Work out the finished part from the listing and answer in its coordinate system (mm). Face numbers are marked on the shaded views. Coordinates: 2 decimals unless noted, no trailing zeros. Loops run counter-clockwise (first coordinate to the right, second up) from the corner with the lowest first, then second, coordinate; pieces in that order, holes last. Notation, with made-up numbers: (51.25, 9) -> (91.25, 9) arc R12 ccw to (91.25, 31) -> close; hole circle Ø4 at (7, 22). An arc over 180 degrees is marked (long way). Answer as CSV lines item,"result".
Autodesk Inventor part; units mm, degrees
ref_plane "Arbeitsebene1" through (2.5, -44.2, -61.269) normal (-1, 0, 0) x (0, 0, 1)
ref_plane "YZ Plane" through (0, 0, 0) normal (1, 0, 0) x (0, 1, 0)
ref_plane "XZ Plane" through (0, 0, 0) normal (0, 1, 0) x (-1, 0, 0)
sketch "Skizze4" plane through (0, 0, 0) normal (1, 0, 0) x (0, 1, 0)
  line L0 (44.5, 24.853) -> (-44.5, 61.718)
  line L1 (-44.5, 61.718) -> (-44.5, -61.718)
  line L2 (-44.5, -61.718) -> (44.5, -24.853)
  line L3 (44.5, -24.853) -> (44.5, 24.853)
  line L4 (0, -86.4052) -> (0, 86.4052) construction
  line L5 (-62.3, 0) -> (62.3, 0) construction
  dimension "d34" = 89
  dimension "d37" = 112.5
  dimension "d38" = 49.706
extrude "Extrusion2" add sketch "Skizze4" along normal blind 2.5
sketch "Skizze5" plane through (2.5, 0, 0) normal (1, 0, 0) x (0, 0, -1)
  line L0 (-61.718, -44.5) -> (61.718, -44.5) construction
  line L1 (61.718, -44.5) -> (24.853, 44.5) construction
  line L2 (24.853, 44.5) -> (-24.853, 44.5) construction
  line L3 (-24.853, 44.5) -> (-61.718, -44.5) construction
  line L4 (-22.8485, 41.5) -> (22.8485, 41.5)
  line L5 (22.8485, 41.5) -> (57.2282, -41.5)
  line L6 (57.2282, -41.5) -> (-57.2282, -41.5)
  line L7 (-57.2282, -41.5) -> (-22.8485, 41.5)
  line L8 (20.8439, 38.5) -> (-20.8439, 38.5)
  line L9 (-20.8439, 38.5) -> (-52.7384, -38.5)
  line L10 (-52.7384, -38.5) -> (52.7384, -38.5)
  line L11 (52.7384, -38.5) -> (20.8439, 38.5)
  point P0 (0, 0)
  dimension "d8" = 3
  dimension "d9" = 3
extrude "Extrusion3" add sketch "Skizze5" along normal blind 3
sketch "Skizze6" plane through (0, 0, 0) normal (-1, 0, 0) x (0, 0, 1)
  line L0 (24.853, 44.5) -> (-24.853, 44.5) construction
  line L1 (61.718, -44.5) -> (24.853, 44.5) construction
  line L2 (-24.853, 44.5) -> (24.853, 44.5)
  line L3 (0, 57.3) -> (0, -53.3) construction
  line L4 (-61.718, -44.5) -> (61.718, -44.5) construction
  arc A0 (-11.1803, -44.5) -> (11.1803, -44.5) centre (0, -34.5) ccw
  line L5 (-11.1803, -44.5) -> (11.1803, -44.5)
  dimension "d35" = 15
  dimension "d36" = 10
extrude "Extrusion4" add sketch "Skizze6" against normal up to surface (2.5 mm away)
sketch "Skizze8" plane through (0, 0, 0) normal (-1, 0, 0) x (0, 0, 1)
  circle A0 centre (0, 56.5) radius 2 construction
  line L0 (-61.718, -44.5) -> (-11.1803, -44.5) construction
  arc A1 (-11.1803, -44.5) -> (11.1803, -44.5) centre (0, -34.5) ccw construction
  line L1 (11.1803, -44.5) -> (61.718, -44.5) construction
  line L2 (61.718, -44.5) -> (24.853, 44.5) construction
  line L3 (24.853, 44.5) -> (-24.853, 44.5) construction
  line L4 (-24.853, 44.5) -> (-61.718, -44.5) construction
  line L5 (0, -71.1) -> (0, 80.1) construction
  line L6 (-86.4052, 0) -> (86.4052, 0) construction
  line L7 (-16.8941, 19.5) -> (16.8941, 19.5) construction
  line L8 (-32.22, -17.5) -> (32.22, -17.5) construction
  line L9 (32.22, -17.5) -> (16.8941, 19.5) construction
  line L10 (-16.8941, 19.5) -> (-32.22, -17.5) construction
  point P0 (0, 0)
  dimension "d42" = 37
  dimension "d53" = 112.5
  dimension "d54" = 25
hole "Bohrung2" at (0, 19.5, -16.8941) at (0, -17.5, -32.22) at (0, -17.5, 32.22) at (0, 19.5, 16.8941) direction (1, 0, 0) diameter 5.4 end through all
chamfer "Fase2" distance 2 angle 45 4 edges at (0, -17.5, -34.92) (0, 19.5, -19.5941) (0, -17.5, 29.52) (0, 19.5, 14.1941)
sketch "Skizze9" plane through (0, 0, 0) normal (-1, 0, 0) x (0, 0, 1)
  line L0 (61.718, -44.5) -> (24.853, 44.5)
  line L1 (11.1803, -44.5) -> (61.718, -44.5)
  line L2 (-61.718, -44.5) -> (-11.1803, -44.5)
  line L3 (-24.853, 44.5) -> (-61.718, -44.5)
  line L4 (24.853, 44.5) -> (-24.853, 44.5)
  line L5 (-11.1803, -44.2) -> (-61.269, -44.2)
  line L6 (-61.269, -44.2) -> (-24.6525, 44.2)
  line L7 (-24.6525, 44.2) -> (24.6525, 44.2)
  line L8 (24.6525, 44.2) -> (61.269, -44.2)
  line L9 (61.269, -44.2) -> (11.1803, -44.2)
  arc A0 (-11.1803, -44.5) -> (11.1803, -44.5) centre (0, -34.5) ccw
  line L10 (11.0454, -44.2) -> (61.269, -44.2)
  line L11 (61.269, -44.2) -> (24.6525, 44.2)
  line L12 (24.6525, 44.2) -> (-24.6525, 44.2)
  line L13 (-24.6525, 44.2) -> (-61.269, -44.2)
  line L14 (-61.269, -44.2) -> (-11.0454, -44.2)
  arc A1 (-11.0454, -44.2) -> (11.0454, -44.2) centre (0, -34.5) ccw
  point P0 (0, 0)
  dimension "d55" = 0.3
  dimension "d56" = 0.3
ref_plane "Arbeitsebene1" through (2.5, -44.2, -61.269) normal (-1, 0, 0) x (0, 0, 1)
extrude "Extrusion5" cut sketch "Skizze9" against normal up to surface (2.5 mm away)
sketch "Skizze10" plane through (0, 0, 0) normal (-1, 0, 0) x (0, 0, 1)
  line L0 (-24.6525, 44.2) -> (-61.269, -44.2) construction
  line L1 (-61.269, -44.2) -> (-11.0454, -44.2) construction
  arc A0 (-11.0454, -44.2) -> (11.0454, -44.2) centre (0, -34.5) ccw construction
  line L2 (11.0454, -44.2) -> (61.269, -44.2) construction
  line L3 (61.269, -44.2) -> (24.6525, 44.2) construction
  line L4 (24.6525, 44.2) -> (-24.6525, 44.2) construction
  circle A1 centre (-32.22, -17.5) radius 4.7 construction
  circle A2 centre (-16.8941, 19.5) radius 4.7 construction
  circle A3 centre (16.8941, 19.5) radius 4.7 construction
  circle A4 centre (32.22, -17.5) radius 4.7 construction
  line L5 (-25.0668, 44.2) -> (25.0668, 44.2)
  line L6 (25.0668, 44.2) -> (25.0668, 43.2)
  line L7 (25.0668, 43.2) -> (-25.0668, 43.2)
  line L8 (-25.0668, 43.2) -> (-25.0668, 44.2)
  line L9 (24.6525, 44.2) -> (-24.6525, 44.2)
  line L10 (24.6525, 44.2) -> (61.269, -44.2)
  point P0 (0, 0)
  dimension "d59" = 1
extrude "Extrusion6" cut sketch "Skizze10" against normal up to surface (2.5 mm away)
fillet "Rundung1" radius 0.5 14 edges at (1.25, 43.2, 25.0668) (1.25, 43.2, -25.0668) (1.25, -44.2, -61.269) (1.25, -44.2, 61.269) (4, -41.5, 57.2282) (4, -41.5, -57.2282) (4, 41.5, -22.8485) (4, 41.5, 22.8485) (4, -38.5, -52.7384) (4, 38.5, -20.8439) (4, 38.5, 20.8439) (4, -38.5, 52.7384) (1.25, -44.2, 11.0454) (1.25, -44.2, -11.0454)
properties part number "Modul Deckel" material "PC/ABS-Kunststoff"
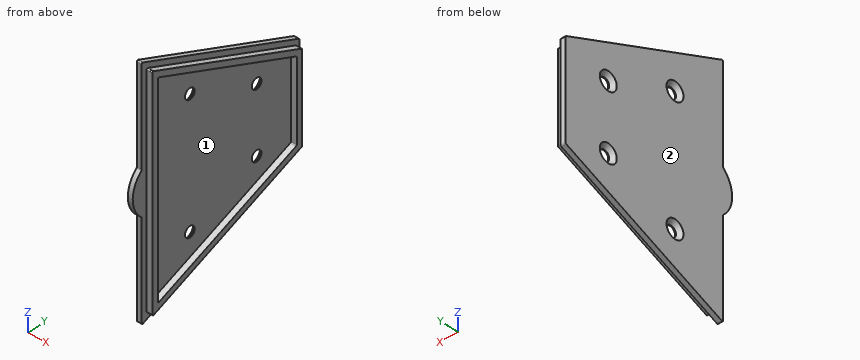
(1) A cutting plane is placed at D-D, the plane y = 34. Write down the section's boundary in (x, z).
Computed values:
outline,"(0, -28.88) -> (2.5, -28.88) -> (2.5, -25.96) -> (5.5, -25.96) -> (5.5, -22.71) -> (2.5, -22.71) -> (2.5, 22.71) -> (5.5, 22.71) -> (5.5, 25.96) -> (2.5, 25.96) -> (2.5, 28.88) -> (0, 28.88) -> close"
(2) A cutting plane is placed at B-B, the plane y = -17.5. Write down the section's boundary in (x, z).
Computed values:
outline,"(0, -50.21) -> (2.5, -50.21) -> (2.5, -47.29) -> (5.5, -47.29) -> (5.5, -44.04) -> (2.5, -44.04) -> (2.5, -34.92) -> (2, -34.92) -> (0, -36.92) -> close; (0, -27.52) -> (2, -29.52) -> (2.5, -29.52) -> (2.5, 29.52) -> (2, 29.52) -> (0, 27.52) -> close; (0, 36.92) -> (2, 34.92) -> (2.5, 34.92) -> (2.5, 44.04) -> (5.5, 44.04) -> (5.5, 47.29) -> (2.5, 47.29) -> (2.5, 50.21) -> (0, 50.21) -> close"
(3) A cutting plane is placed at C-C, the plane z = 32.22. Write down the section's boundary in (x, y).
Computed values:
outline,"(0, -44.2) -> (2.5, -44.2) -> (2.5, -41.5) -> (5.5, -41.5) -> (5.5, -38.5) -> (2.5, -38.5) -> (2.5, -20.2) -> (2, -20.2) -> (0, -22.2) -> close; (0, -12.8) -> (2, -14.8) -> (2.5, -14.8) -> (2.5, 11.04) -> (5.5, 11.04) -> (5.5, 18.88) -> (2.5, 18.88) -> (2.5, 25.93) -> (0, 25.93) -> close"
(4) A cutting plane is placed at A-A, the plane x = 3.85. Write down the section's boundary in (y, z).
Computed values:
outline,"(-41.5, -56.48) arc R0.5 ccw to (-40.81, -56.94) -> (41.19, -22.98) arc R0.5 ccw to (41.5, -22.51) -> (41.5, 22.51) arc R0.5 ccw to (41.19, 22.98) -> (-40.81, 56.94) arc R0.5 ccw to (-41.5, 56.48) -> close; hole (-38.5, -51.99) arc R0.5 ccw to (-37.81, -52.45) -> (38.19, -20.97) arc R0.5 ccw to (38.5, -20.51) -> (38.5, 20.51) arc R0.5 ccw to (38.19, 20.97) -> (-37.81, 52.45) arc R0.5 ccw to (-38.5, 51.99) -> close"
(5) Flat-ended cylindrical pins translate along their axes: pin 1 Ø1.5 at (y, z) = (-22.5, 20.5) entering from -X; pin 2 Ø8.5 at (y, z) = (-17.5, -32.22) entering from -X; pin 3 Ø3 at (x, y) = (2, 33.5) entering from -Z; pin 4 Ø3 at (y, z) = (-17.5, 32.22) entering from -X. Find the tip coordinate at first contact, or state that the pin passes through.
Computed values:
pin 1,"x = 0"
pin 2,"x = 0.45"
pin 3,"z = -29.71"
pin 4,"through"
(6) Consider line 1 along Z through (x, y) = (1.05, 18.5); line 2 along Z through (x, y) = (2.25, 19.5); line 3 along X through (y, z) = (-31, -12). Determine where each line is inside the solid, lowest interval first.
Computed values:
line 1,"-35.3 to -20.4, -13.38 to 13.38, 20.4 to 35.3"
line 2,"-34.88 to -19.59, -14.19 to 14.19, 19.59 to 34.88"
line 3,"0 to 2.5"
(7) For a pull along Z with two mould halves and no side action, classify the marked faces 1 and 2 as pulls with the +Z half, pulls with the -Z half, needs draft (parallel to the pull), parting line crosses it, or undercut.
Computed values:
face 1,"undercut"
face 2,"needs draft"
